```python
from build123d import *

# Parameters (mm, degrees)
FILLET1_R         = 2
CIRPATTERN1_COUNT = 4
SKETCH7_R         = 2.75
EXTRUDE4_DEPTH    = 5.592663071
CHAMFER7_SIZE     = 0.5
CHAMFER7_SIZE2    = 0.288675135
EXTRUDE1_DEPTH    = 1
EXTRUDE2_DEPTH    = 0.375
CIRPATTERN2_COUNT = 2
CIRPATTERN2_ANGLE = 90
CHAMFER8_SIZE     = 0.3
EXTRUDE5_DEPTH    = 4.5
SKETCH10_R        = 0.75
EXTRUDE6_DEPTH    = 1.5


with BuildPart() as part:
    # Sketch1 → Revolve1 (revolve)
    with BuildSketch(Plane.XY):
        with BuildLine():
            Line((4.875, 7.25), (4.875, 11.15))
            add(Edge.make_bspline(
                [(4.875, 11.15), (9.2, 11.15), (9.2, 13.37879152)],
                knots=[0, 0, 0, 1, 1, 1], degree=2))
            add(Edge.make_bspline(
                [(6.5, 15.3), (9.2, 15.3), (9.2, 13.37879152)],
                knots=[0, 0, 0, 1, 1, 1], degree=2))
            ThreePointArc((6.5, 15.3), (3.288236609, 14.551462038), (0, 14.3))
            Line((0, 14.3), (0, 6.592663071))
            Line((0, 6.592663071), (3.625, 6.592663071))
            ThreePointArc((3.625, 6.592663071), (8.487888372, 4.14452152), (12.018330519, 0))
            Line((12.018330519, 0), (13.15, 0))
            ThreePointArc((13.15, 0), (9.714205127, 4.425911714), (4.875, 7.25))
        make_face()
    revolve(axis=Axis((0, 4.818084651, 0), (0, 1, 0)))

    # Fillet1
    fillet1_edges = [part.edges().sort_by_distance(p)[0] for p in [
        (-6.5, 15.3, 0),
    ]]
    fillet(fillet1_edges, radius=FILLET1_R)

    # Sketch2 → Revolve2 (revolve)
    with BuildSketch(Plane.XY):
        with BuildLine():
            Line((5, 15.042457163), (6, 15.042457163))
            ThreePointArc((6, 15.042457163), (5.5, 15.542457163), (5, 15.042457163))
        make_face()
    revolve2 = revolve(axis=Axis((5, 15.042457163, 0), (1, 0, 0)))

    # CirPattern1: Revolve2 ×4 about axis
    cirpattern1_axis = Axis((0, 0, 0), (0, 1, 0))
    for i in range(1, CIRPATTERN1_COUNT):
        add(revolve2.rotate(cirpattern1_axis, i * 360 / CIRPATTERN1_COUNT))

    # Sketch7 → Extrude4 (add)
    with BuildSketch(Plane.XZ.offset(-6.592663071)):
        with Locations(Location((0, 0, 0), (0, 0, 270))):
            Circle(SKETCH7_R)
    extrude(amount=EXTRUDE4_DEPTH)

    # Chamfer7
    chamfer7_edges = [part.edges().sort_by_distance(p)[0] for p in [
        (0, 1, 2.75),
    ]]
    chamfer7_side = [part.faces().sort_by_distance(p)[0] for p in [
        (0, 1, 0),
    ]]
    chamfer(chamfer7_edges, length=CHAMFER7_SIZE, length2=CHAMFER7_SIZE2, reference=chamfer7_side[0])

    # Sketch4 → Extrude1 (add, symmetric)
    with BuildSketch(Plane(origin=(0, 0, 0), x_dir=(-0.7071067811865462, 0, -0.7071067811865488), z_dir=(0.7071067811865488, 0, -0.7071067811865462))):
        with BuildLine():
            Line((-5.5, 5.930708042), (-5.5, 2.488594961))
            Line((-5.5, 2.488594961), (-2.379095763, 1))
            Line((-2.379095763, 1), (2.379095763, 1))
            Line((2.379095763, 1), (5.5, 2.488594961))
            Line((5.5, 2.488594961), (5.5, 5.930708042))
            ThreePointArc((5.5, 5.930708042), (4.574489301, 6.295645476), (3.625, 6.592663071))
            Line((3.625, 6.592663071), (-3.625, 6.592663071))
            ThreePointArc((-3.625, 6.592663071), (-4.574489301, 6.295645476), (-5.5, 5.930708042))
        make_face()
    extrude1 = extrude(amount=EXTRUDE1_DEPTH, both=True)

    # Sketch5 → Extrude2 (add, symmetric)
    with BuildSketch(Plane(origin=(0, 0, 0), x_dir=(0.7071067811865462, 0, 0.7071067811865488), z_dir=(-0.7071067811865488, 0, 0.7071067811865462))):
        with BuildLine():
            Line((-5.5, 2.488594961), (-8.66872656, 4))
            ThreePointArc((-8.66872656, 4), (-7.149832968, 5.072804518), (-5.5, 5.930708042))
            Line((-5.5, 5.930708042), (-5.5, 2.488594961))
        make_face()
        with BuildLine():
            Line((5.5, 2.488594961), (8.66872656, 4))
            ThreePointArc((8.66872656, 4), (7.149832968, 5.072804518), (5.5, 5.930708042))
            Line((5.5, 5.930708042), (5.5, 2.488594961))
        make_face()
    extrude2 = extrude(amount=EXTRUDE2_DEPTH, both=True)

    # CirPattern2: Extrude1, Extrude2 ×2 about axis
    cirpattern2_axis = Axis((0, 0, 0), (0, -1, 0))
    add([extrude1.rotate(cirpattern2_axis, i * CIRPATTERN2_ANGLE / (CIRPATTERN2_COUNT - 1)) for i in range(1, CIRPATTERN2_COUNT)])
    add([extrude2.rotate(cirpattern2_axis, i * CIRPATTERN2_ANGLE / (CIRPATTERN2_COUNT - 1)) for i in range(1, CIRPATTERN2_COUNT)])

    # Chamfer8
    chamfer8_edges = [part.edges().sort_by_distance(p)[0] for p in [
        (-1.682274747, 1, 1.682274747),
        (1.682274747, 1, -1.682274747),
        (1.682274747, 1, 1.682274747),
        (-1.682274747, 1, -1.682274747),
    ]]
    chamfer(chamfer8_edges, length=CHAMFER8_SIZE)

    # Sketch9 → Extrude5 (cut)
    with BuildSketch(Plane.XZ.offset(-1)):
        with BuildLine():
            Line((-1.452368755, 1.375), (-0.375, 1.375))
            ThreePointArc((-0.375, 1.375), (0, 1.544281086), (0.375, 1.375))
            Line((0.375, 1.375), (1.452368755, 1.375))
            ThreePointArc((1.452368755, 1.375), (2, 0), (1.452368755, -1.375))
            Line((1.452368755, -1.375), (-1.452368755, -1.375))
            ThreePointArc((-1.452368755, -1.375), (-2, 0), (-1.452368755, 1.375))
        make_face()
    extrude(amount=-EXTRUDE5_DEPTH, mode=Mode.SUBTRACT)

    # Sketch10 → Extrude6 (cut)
    with BuildSketch(Plane.XZ.offset(-5.5)):
        with Locations(Location((0, 0, 0), (0, 0, 270))):
            Circle(SKETCH10_R)
    extrude(amount=-EXTRUDE6_DEPTH, mode=Mode.SUBTRACT)


solid = part.part
```
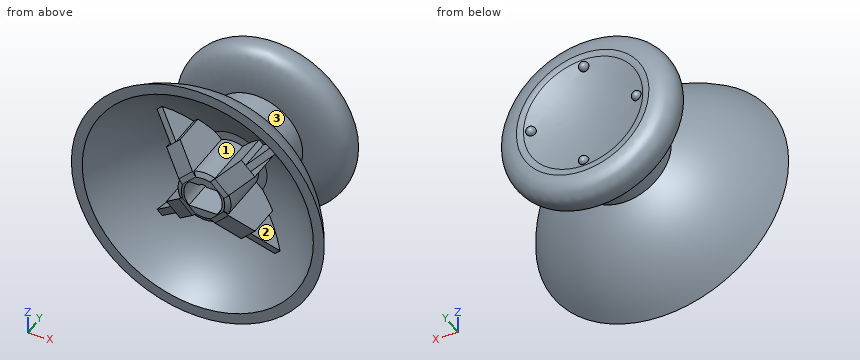
Source: CAD feature listing. Evaluate the final solid. Frame: model axes, mm. Face numbers are marked on the shaded views. Coordinates: 2 decimals unless noted, no trailing zeros. Loops run counter-clockwise (first coordinate to the right, second up) from the corner with the lowest first, then second, coordinate; pieces in that order, holes last. Notation, with made-up numbers: M 79.5,-3 L 133.5,-3 A25 ccw 133.5,27 Z; hole C -4,-6.75 d1. An arc over 180 degrees is marked long. Use a Markdown table: item, result. Add a question column.
Q1. Section query C-C, the plane z = -11. Return loops of the section in (x, y), and give its area (3 significant figures).
Q2. First-contact query: pin 1 (3 mm diameter, centred on x = -5, y = 5, fed in from +Z); pin 2 (1.2 mm diameter, centred on x = -1, y = 2.5, fed in from -Z); pin 3 (8 mm diameter, centred on x = -7.5, y = 6, fed in from +Z). Flat tips, straight axial feed; report the tip coordinate or a pass-through.
Q3. Draft query along X for the marked faces 1, 2 and 3. Return one class per face: pulls with the +X half, pulls with the -X half, needs draft (parallel to the pull), parting line crosses it, or undercut.
Q4. Section query B-B, the plane x = -11. Return loops of the section in (y, z), and give its area (3 significant figures).
Q5. Material intervals for L1, parallel to X at y = 6, z = 0; L2, parallel to X at y = 3.75, z = -1.5; L3, parallel to Y at x = -3.25, z = 7, sorted ascending.
Q6. Section query A-A, the plane y = 3.5. State how many separate pieces and enclosed holes the cut face has, and give its area (3 significant figures).
Result:
| question | item | result |
|---|---|---|
| 1 | outline | M -7.21,0 L -4.84,0 A8.24 cw 4.84,0 L 7.21,0 A9.81 ccw Z |
| 1 | area | 21.0 mm2 |
| 2 | pin 1 | stops at z = 9.6 |
| 2 | pin 2 | stops at z = -11.96 |
| 2 | pin 3 | stops at z = 10.12 |
| 3 | face 1 | undercut |
| 3 | face 2 | undercut |
| 3 | face 3 | parting line crosses it |
| 4 | outline | M 0,-7.21 A9.81 ccw 0,7.21 L 0,4.84 A8.24 cw 0,-4.84 Z |
| 4 | area | 21.0 mm2 |
| 5 | L1 | x = -7.55 to -5.34, -2.75 to -0.75, 0.75 to 2.75, 5.34 to 7.55 |
| 5 | L2 | x = -10.33 to -8.84, -2.91 to 2.91, 8.84 to 10.33 |
| 5 | L3 | y = 4.71 to 5.9, 11.53 to 15.17 |
| 6 | separate pieces | 2 |
| 6 | enclosed holes | 2 |
| 6 | area | 132 mm2 |
